```python
from build123d import *

# Parameters (mm, degrees)
BOSS_EXTRUDE1_DEPTH            = 11.5
CBORE_FOR_M5_SHCS1_D           = 5.3
CBORE_FOR_M5_SHCS1_CBORE_D     = 9.5
CBORE_FOR_M5_SHCS1_CBORE_DEPTH = 10
CHAMFER_2_REACH                = 39.567
SKETCH5_W                      = 48
SKETCH5_H                      = 23
CUT_EXTRUDE2_DEPTH             = 1
CUT_EXTRUDE3_DEPTH             = 38.566607513
CUT_EXTRUDE3_DEPTH_BACK        = 38.566607513
FILLET1_R                      = 1


with BuildPart() as part:
    # Sketch1 → Boss-Extrude1 (new, symmetric)
    with BuildSketch(Plane.XY):
        with BuildLine():
            Line((24, 17.5), (-24, 17.5))
            Line((-24, 17.5), (-24, 0))
            Line((-24, 0), (-16, 0))
            ThreePointArc((-16, 0), (0, 16), (16, 0))
            Line((16, 0), (24, 0))
            Line((24, 0), (24, 17.5))
        make_face()
    extrude(amount=BOSS_EXTRUDE1_DEPTH, both=True)

    # CBORE for M5 SHCS1 (through all)
    with Locations(Plane(origin=(0, 17.5, 0), x_dir=(1, 0, 0), z_dir=(0, 1, 0))):
        with Locations((-19.5, -6), (-19.5, 6), (19.5, -6), (19.5, 6)):
            CounterBoreHole(CBORE_FOR_M5_SHCS1_D / 2, CBORE_FOR_M5_SHCS1_CBORE_D / 2, CBORE_FOR_M5_SHCS1_CBORE_DEPTH)

    # Sketch4 → Chamfer 2 (cut, up to next)
    with BuildSketch(Plane.XY.offset(11.5), mode=Mode.PRIVATE) as chamfer_2_sk1:
        Polygon((24, 17.5), (14, 17.5), (24, 7.5), align=None)
    chamfer_2_tool1 = extrude(chamfer_2_sk1.sketch, amount=-CHAMFER_2_REACH, mode=Mode.PRIVATE) & part.part
    # Sketch4 → Chamfer 2 (cut, up to next)
    with BuildSketch(Plane.XY.offset(11.5), mode=Mode.PRIVATE) as chamfer_2_sk2:
        Polygon((-14, 17.5), (-24, 17.5), (-24, 7.5), align=None)
    chamfer_2_tool2 = extrude(chamfer_2_sk2.sketch, amount=-CHAMFER_2_REACH, mode=Mode.PRIVATE) & part.part
    add(chamfer_2_tool1.solids().sort_by_distance((20.666667, 14.166667, 11.5))[0], mode=Mode.SUBTRACT)
    add(chamfer_2_tool2.solids().sort_by_distance((-20.666667, 14.166667, 11.5))[0], mode=Mode.SUBTRACT)

    # Sketch5 → Cut-Extrude2 (cut)
    with BuildSketch(Plane(origin=(0, 0, 0), x_dir=(-1, 0, 0), z_dir=(0, -1, 0))):
        Rectangle(SKETCH5_W, SKETCH5_H)
    extrude(amount=-CUT_EXTRUDE2_DEPTH, mode=Mode.SUBTRACT)

    # Sketch6 → Cut-Extrude3 (cut, two sides: drawn at the far end of the back side and taken through both)
    with BuildSketch(Plane.XY.offset(11.5).offset(-CUT_EXTRUDE3_DEPTH_BACK)):
        with BuildLine():
            Line((-24, 3.357864376), (-24, 7.5))
            Line((-24, 7.5), (-21.071067812, 10.428932188))
            ThreePointArc((-21.071067812, 10.428932188), (-23.238795325, 7.1846987), (-24, 3.357864376))
        make_face()
        with BuildLine():
            Line((-16.928932188, 14.571067812), (-14, 17.5))
            Line((-14, 17.5), (-9.857864376, 17.5))
            ThreePointArc((-9.857864376, 17.5), (-13.6846987, 16.738795325), (-16.928932188, 14.571067812))
        make_face()
        with BuildLine():
            Line((9.857864376, 17.5), (14, 17.5))
            Line((14, 17.5), (16.928932188, 14.571067812))
            ThreePointArc((16.928932188, 14.571067812), (13.6846987, 16.738795325), (9.857864376, 17.5))
        make_face()
        with BuildLine():
            Line((21.071067812, 10.428932188), (24, 7.5))
            Line((24, 7.5), (24, 3.357864376))
            ThreePointArc((24, 3.357864376), (23.238795325, 7.1846987), (21.071067812, 10.428932188))
        make_face()
    extrude(amount=CUT_EXTRUDE3_DEPTH + CUT_EXTRUDE3_DEPTH_BACK, mode=Mode.SUBTRACT)

    # Fillet1
    fillet1_edges = [part.edges().sort_by_distance(p)[0] for p in [
        (-15.968719423, 1, 0),
        (15.968719423, 1, 0),
        (-24, 1, 0),
        (24, 1, 0),
    ]]
    fillet(fillet1_edges, radius=FILLET1_R)


solid = part.part
```
The model under review builds one solid part; all positions refer to its coordinate system, in mm. A direction names the side the tool comes from. Round coordinates to 2 decimals unless told otherwise and drop trailing zeros. Loops run counter-clockwise (first coordinate to the right, second up) from the corner with the lowest first, then second, coordinate; pieces in that order, holes last. Notation, with made-up numbers: M 51.5,1 L 99.5,1 A18 ccw 99.5,26 Z; hole C -34,-2 d4. An arc over 180 degrees is marked long. Write item = value, one per line.
Item 1: The part is to be moulded in two halves that separate along X. For faces 1 (the flat face through (20, 1, 0)), 2 (the cylindrical face through (16.225, 1.246, -8.919)), 3 (the cylindrical face through (-21.95, 4.2, 7.01)), 4 (the cylindrical face through (-23.699, 1.285, -0.161)), say which applies: released by +X, released by -X, zero draft, split by the parting line, or undercut.
Return value:
face_1 = zero draft
face_2 = undercut
face_3 = undercut
face_4 = released by -X
Item 2: Take a section at D-D on y = 6.5. Write out the cut boundary in (x, z), then the cut area to 3 significant figures.
Return value:
outline = M -23.49,-11.5 L -14.62,-11.5 L -14.62,11.5 L -23.49,11.5 Z; M 14.62,-11.5 L 23.49,-11.5 L 23.49,11.5 L 14.62,11.5 Z; hole C -19.5,-6 d5.3; hole C -19.5,6 d5.3; hole C 19.5,-6 d5.3; hole C 19.5,6 d5.3
area = 320 mm2
Item 3: Take a section at B-B on x = 20. Write out the cut boundary in (y, z).
Return value:
outline = M 1,-11.5 L 11.5,-11.5 L 11.5,-10.72 L 7.5,-10.72 L 7.5,-8.6 L 1,-8.6 Z; M 1,-3.4 L 7.5,-3.4 L 7.5,-1.28 L 11.5,-1.28 L 11.5,1.28 L 7.5,1.28 L 7.5,3.4 L 1,3.4 Z; M 1,8.6 L 7.5,8.6 L 7.5,10.72 L 11.5,10.72 L 11.5,11.5 L 1,11.5 Z
Item 4: Machinability: for faces 5 (the flat face through (17, 7.5, -4)), 6 (the flat face through (-20, 1, 0)), which of the approach directions +Z, -Z, +X, -X, +Y, -Y give a long, thin tool a straight path to every point of the face, cutting with its end or side? Answer none if there is none.
Return value:
face_5 = +Y
face_6 = +Z, -Z, +X, -X, -Y
Item 5: Take a section at A-A on y = 15.5. Write out the cut boundary in (x, z), then the cut area to 3 significant figures.
Return value:
outline = M -15.86,-11.5 L -3.97,-11.5 L -3.97,11.5 L -15.86,11.5 L -15.86,9.05 A4.75 cw -15.86,2.95 L -15.86,-2.95 A4.75 cw -15.86,-9.05 Z; M 3.97,-11.5 L 15.86,-11.5 L 15.86,-9.05 A4.75 cw 15.86,-2.95 L 15.86,2.95 A4.75 cw 15.86,9.05 L 15.86,11.5 L 3.97,11.5 Z
area = 528 mm2
Item 6: Take a section at C-C on y = 2.5. Write out the cut boundary in (x, z), then the cut area to 3 significant figures.
Return value:
outline = M -24,-11.5 L -15.8,-11.5 L -15.8,11.5 L -24,11.5 Z; M 15.8,-11.5 L 24,-11.5 L 24,11.5 L 15.8,11.5 Z; hole C -19.5,-6 d5.3; hole C -19.5,6 d5.3; hole C 19.5,-6 d5.3; hole C 19.5,6 d5.3
area = 289 mm2
Item 7: Insertion check: P1, Ø4, axis at x = -19.5, z = 6, coming from the -Y side; P2, Ø2.5, axis at x = -17, z = -8, coming from the +Y side; P3, Ø1, axis at y = 14, z = 0, coming from the -X side; P4, Ø6, axis at x = -1.5, z = -8, coming from the -Y side. Each pin has a flat end and moves straight along its axis. Give the tip position at first contact, or say it passes through.
Return value:
P1 = through
P2 = 7.5
P3 = -18
P4 = 15.35
Item 8: For line 1 (Z direction, x = 19.5, y = 9.75); line 2 (Z direction, x = 19.5, y = 4.75); line 3 (X direction, y = 8.5, z = 2), list the stretches that pass through material, from the lowest coordinate up. Write a range as [from, to].
Return value:
line_1 = [-11.5, -10.75], [-1.25, 1.25], [10.75, 11.5]
line_2 = [-11.5, -8.65], [-3.35, 3.35], [8.65, 11.5]
line_3 = [-22.58, -22.06], [-16.94, -13.56], [13.56, 16.94], [22.06, 22.58]
